Model file for the job. Use its own axes, mm. A direction names the side the tool comes from. Give positions to 0.01 mm unless a question says otherwise; leave off trailing zeros. Write each loop counter-clockwise with the first axis right and the second up, starting at its lowest first coordinate (ties: lowest second). Pieces come first, ordered by that corner, then holes. Notation, with made-up numbers: (25.25, -16) - (45.25, -16) arc R19 ccw to (45.25, 21) - close; hole circle Ø5 at (-25, -28.5). An arc over 180 degrees is marked (long way). One line per item, written item: value. Start each with the question number.
(1) Probe L1, parallel to X at y = 18.5, z = -11.5; L2, parallel to Y at x = 163.5, z = -11.25; L3, parallel to Y at x = 289, z = -16.25. List the from-to ranges inside material, lowest first.
(2) 3-axis set-ups, long thin cutter, end or side, ignore diameter. For faces 1 (the face through (88.9, 13, -10)), 2 (the face through (288, 129, -10)), 3 (the face through (288, 52, -20)): which of +Z, -Z, +X, -X, +Y, -Y reach the whole face in a straight line?
(3) Cut at C-C, the plane x = 505.5. List the corners of the cut face in (y, z), and give its area (3 significant figures).
(4) Cut at B-B, the plane x = 159. List the corners of the cut face in (y, z).
(5) Drop flat-ended pins along their axis: P1, Ø6, axis at x = 169.5, z = -14.5, coming from the +Y side; P2, Ø1, axis at x = 521, y = 61, coming from the +Z side. Give the stop position or say it passes through.
(6) Cut at A-A, the plane z = -14.5. List the corners of the cut face in (x, y).
(7) Cut at D-D, the plane y = 125.5. List the corners of the cut face in (x, z).
(8) Mould opens along X. For faces 4 (the face through (0, 59, -10)), 5 (the face through (288, 101.6, -15)), 6 (the face through (368.7, 13, -10)) say: pulls with the +X half, pulls with the -X half, needs draft (parallel to the pull), parting line crosses it, or undercut.
Autodesk Inventor part; units mm, degrees
ref_plane "Work Plane2" through (609.4222, 0, -20) normal (0, 0, -1) x (-1, 0, 0)
ref_plane "Work Plane1" through (609.4222, 0, -20) normal (0, 0, -1) x (-1, 0, 0)
ref_plane "YZ Plane" through (0, 0, 0) normal (1, 0, 0) x (0, 1, 0)
sketch "Sketch1" plane through (0, 0, 0) normal (1, 0, 0) x (0, 1, 0)
  line L0 (0, 0) -> (155.1, 0)
  line L1 (155.1, 0) -> (155.1, -10)
  line L2 (0, -20) -> (0, 0)
  line L3 (155.1, -10) -> (101.6, -10)
  line L4 (101.6, -10) -> (101.6, -20)
  line L5 (101.6, -20) -> (0, -20)
  dimension "d0" = 53.5
  dimension "d1" = 155.1
  dimension "d2" = 10
  dimension "d3" = 10
  dimension "d4" = 20
extrude "Extrusion1" add sketch "Sketch1" along normal blind 584.6
ref_plane "Work Plane2" through (609.4222, 0, -20) normal (0, 0, -1) x (-1, 0, 0)
sketch "Sketch2" plane through (609.4222, 0, -20) normal (0, 0, -1) x (-1, 0, 0)
  line L0 (609.4222, 0) -> (609.4222, 155.1)
  line L1 (609.4222, 0) -> (609.4222, 6.35)
  line L2 (520.5222, 6.35) -> (520.5222, 19.05)
  line L3 (520.5222, 19.05) -> (393.1222, 19.05)
  line L4 (393.1222, 19.05) -> (393.1222, 6.35)
  line L5 (393.1222, 6.35) -> (240.7222, 6.35)
  line L6 (240.7222, 6.35) -> (240.7222, 19.05)
  line L7 (240.7222, 19.05) -> (113.7222, 19.05)
  line L8 (113.7222, 19.05) -> (113.7222, 6.35)
  line L9 (113.7222, 6.35) -> (240.7222, 6.35)
  line L10 (393.1222, 6.35) -> (520.5222, 6.35)
  line L11 (24.8222, 0) -> (24.8222, 101.6)
  dimension "d39" = 6.35
  dimension "d41" = 12.7
  dimension "d42" = 90
  dimension "d43" = 152.4
  dimension "d44" = 127
  dimension "d45" = 12.7
  dimension "d58" = 88.9
ref_plane "Work Plane1" through (609.4222, 0, -20) normal (0, 0, -1) x (-1, 0, 0)
sketch "Sketch3" plane through (609.4222, 0, -20) normal (0, 0, -1) x (-1, 0, 0)
  line L0 (609.4222, 0) -> (609.4222, 155.1)
  line L1 (609.4222, 0) -> (609.4222, 6.35)
  line L2 (520.5222, 6.35) -> (520.5222, 19.05)
  line L3 (520.5222, 19.05) -> (393.1222, 19.05)
  line L4 (393.1222, 19.05) -> (393.1222, 6.35)
  line L5 (393.1222, 6.35) -> (240.7222, 6.35)
  line L6 (240.7222, 6.35) -> (240.7222, 19.05)
  line L7 (240.7222, 19.05) -> (113.7222, 19.05)
  line L8 (113.7222, 19.05) -> (113.7222, 6.35)
  line L9 (113.7222, 6.35) -> (240.7222, 6.35)
  line L10 (393.1222, 6.35) -> (520.5222, 6.35)
  line L11 (24.8222, 0) -> (24.8222, 101.6)
  dimension "d46" = 6.35
  dimension "d48" = 12.7
  dimension "d49" = 90
  dimension "d50" = 152.4
  dimension "d51" = 127
  dimension "d52" = 12.7
  dimension "d57" = 88.9
extrude "Extrusion4" cut sketch "Sketch3" against normal blind 127 contours L9 L8 L7 L6
extrude "Extrusion5" cut sketch "Sketch2" against normal blind 127 contours L10 L4 L3 L2
properties part number "SkinnySideW" material "Wood (Birch)"
Answers follow:
1. L1: x = 0 to 88.9, 216.3 to 368.7, 495.7 to 584.6
1. L2: y = 0 to 6.35, 19.05 to 101.6
1. L3: y = 0 to 101.6
2. face 1: +Z, -Z
2. face 2: -Z, +X, -X, +Y
2. face 3: -Z, +X, -X, +Y, -Y
3. outline: (0, -20) - (101.6, -20) - (101.6, -10) - (155.1, -10) - (155.1, 0) - (0, 0) - close
3. area: 2,570 mm²
4. outline: (0, -20) - (6.35, -20) - (6.35, 0) - (0, 0) - close; (19.05, -20) - (101.6, -20) - (101.6, -10) - (155.1, -10) - (155.1, 0) - (19.05, 0) - close
5. P1: stops at y = 101.6
5. P2: stops at z = 0
6. outline: (0, 0) - (584.6, 0) - (584.6, 101.6) - (0, 101.6) - close; hole (88.9, 6.35) - (216.3, 6.35) - (216.3, 19.05) - (88.9, 19.05) - close; hole (368.7, 6.35) - (495.7, 6.35) - (495.7, 19.05) - (368.7, 19.05) - close
7. outline: (0, -10) - (584.6, -10) - (584.6, 0) - (0, 0) - close
8. face 4: pulls with the -X half
8. face 5: needs draft
8. face 6: undercut
